```python
from build123d import *

# Parameters (mm, degrees)
SKETCH003_W            = 20
SKETCH003_H            = 27
PAD001_DEPTH           = 50
SKETCH004_W            = 10
SKETCH004_H            = 2
POCKET002_DEPTH        = 20.001
LINEARPATTERN002_COUNT = 4
LINEARPATTERN002_PITCH = 12
SKETCH005_W            = 2
SKETCH005_H            = 20
POCKET003_DEPTH        = 15
LINEARPATTERN003_COUNT = 2
LINEARPATTERN003_PITCH = 26


with BuildPart() as part:
    # Sketch003 (on ShapeBinder) → Pad001 (new body)
    with BuildSketch(Plane(origin=(0, 0, 0), x_dir=(-1, 0, 0), z_dir=(0, 1, 0))):
        with Locations((-15.8, 19.3)):
            Rectangle(SKETCH003_W, SKETCH003_H)
    extrude(amount=PAD001_DEPTH)

    # Sketch004 (on Face2 of Pad001) → Pocket002 (cut, through all)
    with BuildSketch(Plane(origin=(5.8, 0, 0), x_dir=(0, -1, 0), z_dir=(-1, 0, 0))):
        with Locations((-7, 7.6)):
            Rectangle(SKETCH004_W, SKETCH004_H)
    pocket002 = extrude(amount=-POCKET002_DEPTH, mode=Mode.SUBTRACT)

    # LinearPattern002: Pocket002 ×4
    with Locations(*[(0, i * LINEARPATTERN002_PITCH, 0) for i in range(1, LINEARPATTERN002_COUNT)]):
        add(pocket002, mode=Mode.SUBTRACT)

    # Sketch005 (on Face1 of LinearPattern002) → Pocket003 (cut)
    with BuildSketch(Plane.XY.offset(32.8)):
        with Locations((7.6, 12)):
            Rectangle(SKETCH005_W, SKETCH005_H)
        with Locations((24, 12)):
            Rectangle(SKETCH005_W, SKETCH005_H)
    pocket003 = extrude(amount=-POCKET003_DEPTH, mode=Mode.SUBTRACT)

    # LinearPattern003: Pocket003 ×2
    with Locations(*[(0, i * LINEARPATTERN003_PITCH, 0) for i in range(1, LINEARPATTERN003_COUNT)]):
        add(pocket003, mode=Mode.SUBTRACT)


solid = part.part
```
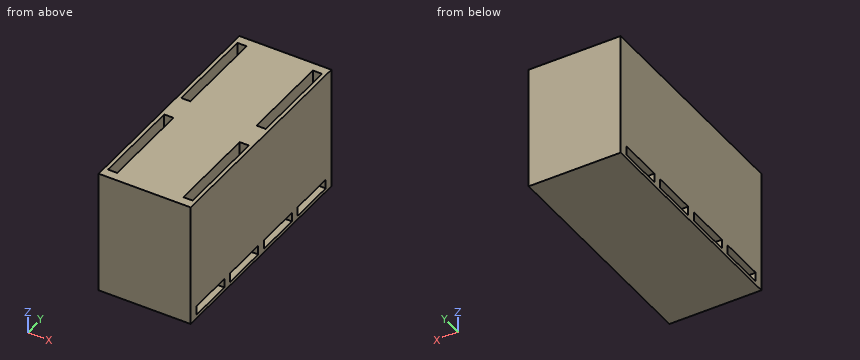
Here's how the part is built. I have some questions about the finished solid (model axes, mm). Give positions to 0.01 mm unless a question says otherwise; leave off trailing zeros. Write each loop counter-clockwise with the first axis right and the second up, starting at its lowest first coordinate (ties: lowest second). Pieces come first, ordered by that corner, then holes.
(1) If I drill on L1, parallel to X at y = 31, z = 23; L2, parallel to Z at x = 17.5, y = 44.5; L3, parallel to Y at x = 8.5, z = 27.5, over which ranges is the centre line in solid material (lowest first)?
Output values:
L1: x = 5.8 to 6.6, 8.6 to 23, 25 to 25.8
L2: z = 5.8 to 6.6, 8.6 to 32.8
L3: y = 0 to 2, 22 to 28, 48 to 50
(2) Imagine slicing it at B-B, the plane x = 24. Write out the boundary of the cut face in (y, z), and give its area (3 significant figures).
Output values:
outline: (0, 5.8) - (50, 5.8) - (50, 32.8) - (48, 32.8) - (48, 17.8) - (28, 17.8) - (28, 32.8) - (22, 32.8) - (22, 17.8) - (2, 17.8) - (2, 32.8) - (0, 32.8) - close; hole (2, 6.6) - (12, 6.6) - (12, 8.6) - (2, 8.6) - close; hole (14, 6.6) - (24, 6.6) - (24, 8.6) - (14, 8.6) - close; hole (26, 6.6) - (36, 6.6) - (36, 8.6) - (26, 8.6) - close; hole (38, 6.6) - (48, 6.6) - (48, 8.6) - (38, 8.6) - close
area: 670 mm2
(3) Imagine slicing it at A-A, the plane y = 21.5. Write out the boundary of the cut face in (x, z).
Output values:
outline: (5.8, 5.8) - (25.8, 5.8) - (25.8, 6.6) - (5.8, 6.6) - close; (5.8, 8.6) - (25.8, 8.6) - (25.8, 32.8) - (25, 32.8) - (25, 17.8) - (23, 17.8) - (23, 32.8) - (8.6, 32.8) - (8.6, 17.8) - (6.6, 17.8) - (6.6, 32.8) - (5.8, 32.8) - close
(4) Imagine slicing it at C-C, the plane z = 29.25. Write out the boundary of the cut face in (x, y), and give its area (3 significant figures).
Output values:
outline: (5.8, 0) - (25.8, 0) - (25.8, 50) - (5.8, 50) - close; hole (6.6, 2) - (8.6, 2) - (8.6, 22) - (6.6, 22) - close; hole (6.6, 28) - (8.6, 28) - (8.6, 48) - (6.6, 48) - close; hole (23, 2) - (25, 2) - (25, 22) - (23, 22) - close; hole (23, 28) - (25, 28) - (25, 48) - (23, 48) - close
area: 840 mm2
(5) Imagine slicing it at D-D, the plane z = 7.5. Write out the boundary of the cut face in (x, y), and give its area (3 significant figures).
Output values:
outline: (5.8, 0) - (25.8, 0) - (25.8, 2) - (5.8, 2) - close; (5.8, 12) - (25.8, 12) - (25.8, 14) - (5.8, 14) - close; (5.8, 24) - (25.8, 24) - (25.8, 26) - (5.8, 26) - close; (5.8, 36) - (25.8, 36) - (25.8, 38) - (5.8, 38) - close; (5.8, 48) - (25.8, 48) - (25.8, 50) - (5.8, 50) - close
area: 200 mm2
(6) Will these pins go through, and if not, where does the flat tip stop? pin 1 (0.6 mm diameter, centred on x = 23.5, z = 28, fed in from -Y); pin 2 (0.6 mm diameter, centred on x = 24, y = 35, fed in from +Z).
Output values:
pin 1: stops at y = 0
pin 2: stops at z = 17.8
